Answer from the drawing. Dimensions are ordinates in mm from the lowest x, y and z of the part. Coordinates: 2 decimals unless noted, no trailing zeros. Order: outer loops, then holes, each group sorted by start corner. A loop starts at its lowest first (then second) coordinate and runs counter-clockwise, first axis right, second up. Notation, with made-up numbers: M -23,76.25 L -18,76.25 A17 cw -18,108.25 Z; hole C 83.5,18.25 d7. An arc over 180 degrees is marked long. One line per question, with ' | ' between items. Start each with the question number.
1) Consider probe 1 along Z at (x, y) = (21.25, 0.8); probe 2 along Z at (x, y) = (17.5, 0.45). Determine where each line is inside the solid, lowest interval first.
2) Find section A-A, the plane z = 90.5. Write down the section's boundary in (x, y).
3) Find section C-C, the plane y = 0.5. Count the separate pieces of the cut face and the enclosed holes in it, plus the area to 3 significant figures.
4) Find section B-B, the plane x = 16.5. Write down the section's boundary in (y, z).
5) Given P1, Ø9, axis at x = 6.26, z = 90.5, coming from the +Y side, flat-ended and moving along its own axis, determine where the tip first touches the part or whether it passes through.
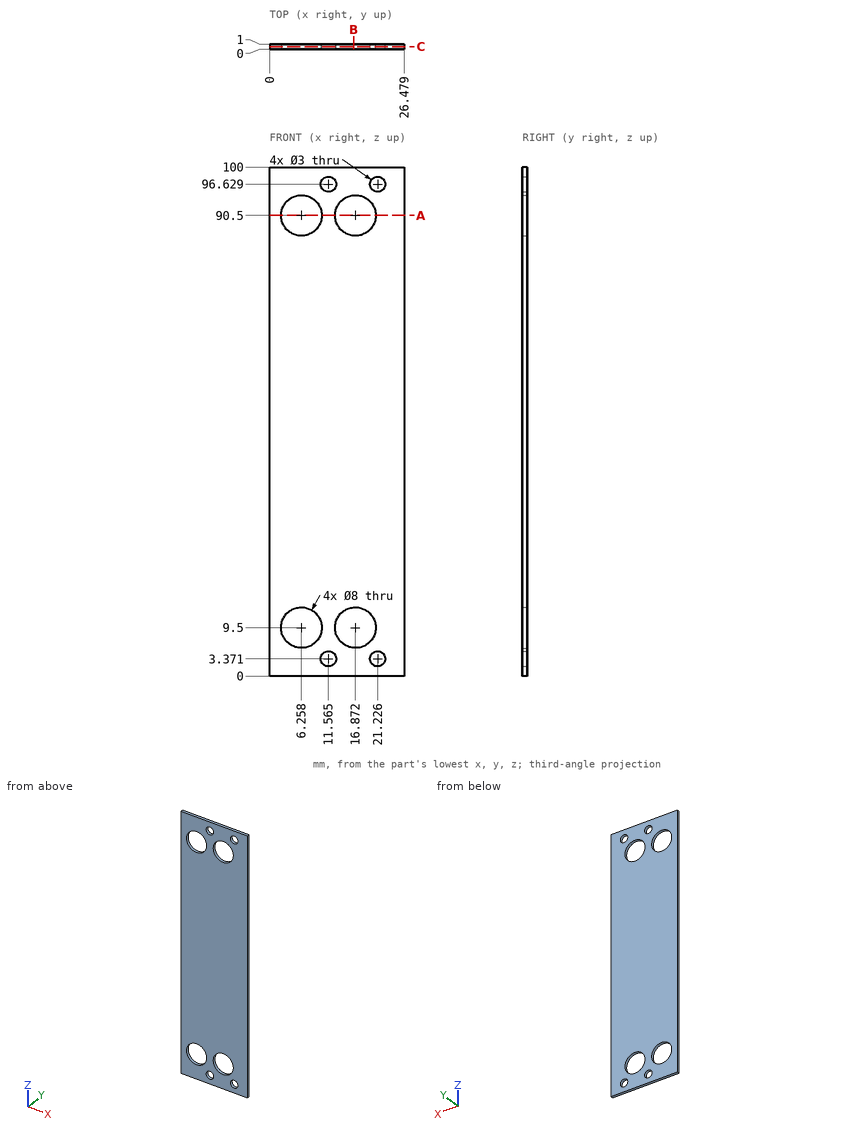
Report:
1) probe 1: z = 0 to 1.87, 4.87 to 95.13, 98.13 to 100 | probe 2: z = 0 to 5.55, 13.45 to 86.55, 94.45 to 100
2) outline: M 0,0 L 2.26,0 L 2.26,1 L 0,1 Z; M 10.26,0 L 12.87,0 L 12.87,1 L 10.26,1 Z; M 20.87,0 L 26.48,0 L 26.48,1 L 20.87,1 Z
3) separate pieces: 1 | enclosed holes: 8 | area: 2,420 mm^2
4) outline: M 0,0 L 1,0 L 1,5.52 L 0,5.52 Z; M 0,13.48 L 1,13.48 L 1,86.52 L 0,86.52 Z; M 0,94.48 L 1,94.48 L 1,100 L 0,100 Z
5) P1: stops at y = 1
